from build123d import *

# Parameters (mm, degrees)
F0_W     = 76.2
F0_H     = 50.8
F0_R     = 12.7
F1_DEPTH = 12.7
F2_W     = 6.35
F2_H     = 50.8
F3_DEPTH = 2.54
F5_DEPTH = 65.278
F6_R     = 4.7625
F7_DEPTH = 12.7


with BuildPart() as f1:
    # F0 (on Top) → F1 (new body)
    with BuildSketch(Plane.XY):
        Rectangle(F0_W, F0_H)
        Circle(F0_R, mode=Mode.SUBTRACT)
    extrude(amount=F1_DEPTH)

    # F2 (on face) → F3 (cut)
    with BuildSketch(Plane.XY.offset(12.7)):
        with Locations((-32.385, 0)):
            Rectangle(F2_W, F2_H)
        with BuildLine():
            Line((6.35, 25.4), (-6.35, 25.4))
            Line((-6.35, 25.4), (-6.35, 10.9985226281))
            ThreePointArc((-6.35, 10.9985226281), (0, 12.7), (6.35, 10.9985226281))
            Line((6.35, 10.9985226281), (6.35, 25.4))
        make_face()
        with BuildLine():
            Line((-6.35, -10.9985226281), (-6.35, -25.4))
            Line((-6.35, -25.4), (6.35, -25.4))
            Line((6.35, -25.4), (6.35, -10.9985226281))
            ThreePointArc((6.35, -10.9985226281), (0, -12.7), (-6.35, -10.9985226281))
        make_face()
    extrude(amount=-F3_DEPTH, mode=Mode.SUBTRACT)

    # F4 (on face) → F5 (cut)
    with BuildSketch(Plane.XZ.offset(25.4)):
        Polygon((28.575, 12.7), (22.225, 12.7), (19.2920606325, 7.62), (31.5079393675, 7.62), align=None)
    extrude(amount=-F5_DEPTH, mode=Mode.SUBTRACT)

    # F6 (on face) → F7 (join)
    with BuildSketch(Plane.YZ.offset(38.1)):
        with Locations((0, 6.35)):
            Circle(F6_R)
    extrude(amount=F7_DEPTH)


solid = f1.part
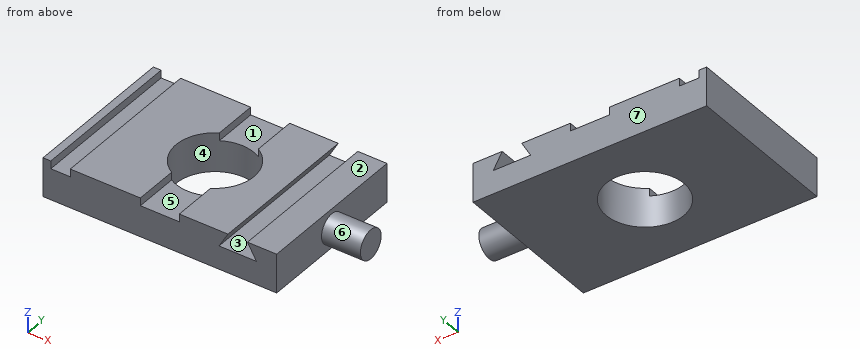
Can you work these out from the model? Positions are in its coordinate system, mm. Face numbers are marked on the shaded views. A direction names the side the tool comes from. Round coordinates to 2 decimals unless told otherwise and drop trailing zeros. Loops run counter-clockwise (first coordinate to the right, second up) from the corner with the lowest first, then second, coordinate; pieces in that order, holes last. Notation, with made-up numbers: (1.25, 42) - (7.25, 42) arc R33 ccw to (7.25, 80) - close; hole circle Ø6 at (28, 2.25). An arc over 180 degrees is marked (long way). Write item = value, one per line. Start each with the question number.
(1) If we mould it in two halves opening along Y, with no side actions, what happens to the marked faces 4, 5, 6 and 7? For each: released by +Y, released by -Y, zero draft, split by the parting line, or undercut.
(2) If we section it at A-A (y = 0): Please give me the cut outline in (x, z) (1 decimal), and give its area (3 significant figures).
(3) If I drill on probe 1 along X at (y, z) = (0, 3.75); probe 2 along Y at (x, z) = (0, 9); probe 3 along X at (y, z) = (0, 9.25), over which ranges is the centre line in solid material (lowest first)? Write a range as [from, to].
(4) If we section it at B-B (z = 6.35): Please give me the cut outline in (x, y), and give its area (3 significant figures).
(5) If we section it at C-C (x = 0): Please give me the cut outline in (y, z), and give its area (3 significant figures).
(6) For P1, Ø1.3, axis at y = -11, z = 11, coming from the +X side; P2, Ø20.5, axis at x = 0, y = 0, coming from the -Z side; P3, Ø3, axis at x = 40, z = 4, coming from the +Y side; P4, Ø3, axis at x = -31.5, y = 0, coming from the +Z side, each with a flat end and sliding along its axis, tell me the tip position at first contact or that it passes through.
(7) For the marked faces 1, 2 and 3, which set-ups out of +Z, -Z, +X, -X, +Y, -Y let a thin tool reach every point of the face, with its end or its side?
(8) If we section it at D-D (y = 18): Please give me the cut outline in (x, z) (3 decimals).
Ans:
q1.face_4 = undercut
q1.face_5 = zero draft
q1.face_6 = split by the parting line
q1.face_7 = released by +Y
q2.outline = (-38.1, 0) - (-12.7, 0) - (-12.7, 12.7) - (-29.2, 12.7) - (-29.2, 10.2) - (-35.6, 10.2) - (-35.6, 12.7) - (-38.1, 12.7) - close; (12.7, 0) - (38.1, 0) - (38.1, 1.6) - (50.8, 1.6) - (50.8, 11.1) - (38.1, 11.1) - (38.1, 12.7) - (28.6, 12.7) - (31.5, 7.6) - (19.3, 7.6) - (22.2, 12.7) - (12.7, 12.7) - close
q2.area = 703 mm²
q3.probe_1 = [-38.1, -12.7], [12.7, 50.8]
q3.probe_2 = [-25.4, -12.7], [12.7, 25.4]
q3.probe_3 = [-38.1, -12.7], [12.7, 20.23], [30.57, 50.8]
q4.outline = (-38.1, -25.4) - (38.1, -25.4) - (38.1, -4.76) - (50.8, -4.76) - (50.8, 4.76) - (38.1, 4.76) - (38.1, 25.4) - (-38.1, 25.4) - close; hole circle Ø25.4 at (0, 0)
q4.area = 3,490 mm²
q5.outline = (-25.4, 0) - (-12.7, 0) - (-12.7, 10.16) - (-25.4, 10.16) - close; (12.7, 0) - (25.4, 0) - (25.4, 10.16) - (12.7, 10.16) - close
q5.area = 258 mm²
q6.P1 = 38.1
q6.P2 = through
q6.P3 = 4.69
q6.P4 = 10.16
q7.face_1 = +Z, +Y, -Y
q7.face_2 = +Z, +X, -X, +Y, -Y
q7.face_3 = +Y, -Y
q8.outline = (-38.1, 0) - (38.1, 0) - (38.1, 12.7) - (28.575, 12.7) - (31.508, 7.62) - (19.292, 7.62) - (22.225, 12.7) - (6.35, 12.7) - (6.35, 10.16) - (-6.35, 10.16) - (-6.35, 12.7) - (-29.21, 12.7) - (-29.21, 10.16) - (-35.56, 10.16) - (-35.56, 12.7) - (-38.1, 12.7) - close
